The listing builds one solid part. Answer for the finished solid, in the listing's coordinates (mm). A direction names the side the tool comes from. Round coordinates to 2 decimals unless told otherwise and drop trailing zeros. Write each loop counter-clockwise with the first axis right and the second up, starting at its lowest first coordinate (ties: lowest second). Pieces come first, ordered by that corner, then holes.
(1) For faces 1 (the face through (17, 25.4, 8)), 2 (the face through (-9, -17, 9.525)), 3 (the face through (22.225, 17, 18)), 4 (the face through (41.275, 0, 8)), 5 (the face through (-41.275, 0, 0)), determine the directions among +Z, -Z, +X, -X, +Y, -Y from which every point of the face is accessible in a straight line to the end or side of a thin tool.
(2) Find the intervals of material crossed by probe 1 along Y at (x, z) = (16.5, 36); probe 2 along Z at (x, y) = (22, 9) (3 decimals); probe 3 along X at (y, z) = (16.5, 8) (3 decimals), in increasing order.
(3) A cutting plane is placed at A-A, the plane z = -2.5. Give the vertices of the cut face in (x, y) (3 decimals).
(4) Each of these flat-tipped pins is pushed along its axis until it touches: pin 1 Ø2.5 at (x, y) = (59.5, -7) entering from -Z; pin 2 Ø8.5 at (y, z) = (20, 18) entering from -X (3 decimals); pin 3 Ø1 at (x, y) = (49, 5) entering from -Z. Where does it stop, or does it pass through?
from build123d import *

# Parameters (mm, degrees)
F1_DEPTH = 25.4
F2_DEPTH = 7.9375


with BuildPart() as f1:
    # F0 (on Front) → F1 (new body, symmetric)
    with BuildSketch(Plane.XZ):
        Polygon((22.225, 9.525), (-41.275, 9.525), (-41.275, -9.525), (41.275, -9.525), (41.275, 9.525), align=None)
        with BuildLine():
            Line((22.225, 27.0002), (22.225, 9.525))
            Line((22.225, 9.525), (41.275, 9.525))
            Line((41.275, 9.525), (41.275, 27.0002))
            ThreePointArc((41.275, 27.0002), (45.92468, 38.22552), (57.15, 42.8752))
            Line((57.15, 42.8752), (60.325, 42.8752))
            Line((60.325, 42.8752), (60.325, 61.9252))
            Line((60.325, 61.9252), (57.15, 61.9252))
            add(Edge.make_bspline(
                [(56.829578, 61.92373), (56.936552, 61.924385), (57.04336, 61.924875), (57.15, 61.9252)],
                knots=[111.193178, 111.193178, 111.193178, 111.193178, 111.504536, 111.504536, 111.504536, 111.504536], degree=3))
            ThreePointArc((56.829578, 61.92373), (32.341268, 51.582357), (22.225, 27.0002))
        make_face()
    extrude(amount=F1_DEPTH, both=True)

    # F0 (on Front) → F2 (join, symmetric)
    with BuildSketch(Plane.XZ):
        with BuildLine():
            add(Edge.make_bspline(
                [(-41.275, 9.525), (-40.764818, 40.487092), (18.626642, 61.690006), (56.829578, 61.92373)],
                knots=[0, 0, 0, 0, 111.193178, 111.193178, 111.193178, 111.193178], degree=3))
            Line((-41.275, 9.525), (22.225, 9.525))
            Line((22.225, 9.525), (22.225, 27.0002))
            ThreePointArc((22.225, 27.0002), (32.341268, 51.582357), (56.829578, 61.92373))
        make_face()
    extrude(amount=F2_DEPTH, both=True)


solid = f1.part
Solutions:
1. face 1: +Z, -Z, +X, -X, +Y
1. face 2: +Z, -X, -Y
1. face 3: +Z, -X, +Y
1. face 4: -Z, +X, +Y, -Y
1. face 5: +Z, -Z, -X, +Y, -Y
2. probe 1: y = -7.94 to 7.94
2. probe 2: z = -9.525 to 9.525
2. probe 3: x = -41.275 to 41.275
3. outline: (-41.275, -25.4) - (41.275, -25.4) - (41.275, 25.4) - (-41.275, 25.4) - close
4. pin 1: stops at z = 42.88
4. pin 2: stops at x = 22.225
4. pin 3: stops at z = 40.31
